from build123d import *

# Parameters (mm, degrees)
BOSS_EXTRUDE2_DEPTH = 2
SKETCH8_R           = 0.46
CUT_EXTRUDE1_DEPTH  = 6.857687257
CUT_EXTRUDE3_DEPTH  = 5.308421985
BOSS_EXTRUDE3_DEPTH = 0.75
SKETCH11_W          = 5.5
SKETCH11_H          = 5
BOSS_EXTRUDE4_DEPTH = 0.75
FILLET1_R           = 2
CUT_EXTRUDE5_DEPTH  = 1.75
SKETCH13_W          = 0.75
SKETCH13_H          = 1.75
CUT_EXTRUDE4_DEPTH  = 0.5
FILLET2_R           = 0.25
FILLET3_R           = 0.25
SKETCH15_RX         = 1.5
SKETCH15_RY         = 0.25
CUT_EXTRUDE6_DEPTH  = 10


with BuildPart() as part:
    # Sketch5 → Boss-Extrude2 (new body)
    with BuildSketch(Plane(origin=(0, 0, 0), x_dir=(1, 0, 0), z_dir=(0, 1, 0))):
        Polygon((-2.25, -2), (1.75, -2), (3.25, -2), (3.25, 2), (1.75, 2), (-2.25, 2), align=None)
    extrude(amount=-BOSS_EXTRUDE2_DEPTH)

    # Sketch8 → Cut-Extrude1 (cut, through all)
    with BuildSketch(Plane(origin=(0.85, 2.55, 0), x_dir=(0.948683298050514, -0.3162277660168378, 0), z_dir=(0.3162277660168378, 0.948683298050514, 0))):
        with Locations((1.829822128, 0)):
            Circle(SKETCH8_R)
    extrude(amount=-CUT_EXTRUDE1_DEPTH, mode=Mode.SUBTRACT)

    # Sketch12 → Cut-Extrude3 (cut, through all)
    with BuildSketch(Plane(origin=(0, 0, 0), x_dir=(1, 0, 0), z_dir=(0, 1, 0))):
        Polygon((-1.5, 1.25), (-1.5, -1.25), (-0.75, -1.25), (0, 0), (-0.75, 1.25), align=None)
    extrude(amount=-CUT_EXTRUDE3_DEPTH, mode=Mode.SUBTRACT)

    # Sketch10 → Boss-Extrude3 (add)
    with BuildSketch(Plane.XY.offset(2)):
        Polygon((3.25, -2), (3.25, 3), (-2.25, 3), (-2.25, 0), (-2.25, -2), align=None)
    boss_extrude3 = extrude(amount=BOSS_EXTRUDE3_DEPTH)

    # Mirror1: Boss-Extrude3 across plane
    add(boss_extrude3.mirror(Plane.XY))

    # Sketch11 → Boss-Extrude4 (add)
    with BuildSketch(Plane(origin=(3.25, 0, 0), x_dir=(0, 0, -1), z_dir=(1, 0, 0))):
        with Locations((0, 0.5)):
            Rectangle(SKETCH11_W, SKETCH11_H)
    extrude(amount=BOSS_EXTRUDE4_DEPTH)

    # Fillet1
    fillet1_edges = [part.edges().sort_by_distance(p)[0] for p in [
        (-2.25, 3, 2.375),
        (-2.25, 3, -2.375),
    ]]
    fillet(fillet1_edges, radius=FILLET1_R)

    # Sketch14 → Cut-Extrude5 (cut)
    with BuildSketch(Plane.XZ.offset(2)):
        Polygon((-2.25, 2.75), (-2.25, 2.25), (3.5, 2.25), (3.5, -2.25), (-2.25, -2.25), (-2.25, -2.75), (4, -2.75), (4, 2.75), align=None)
    extrude(amount=-CUT_EXTRUDE5_DEPTH, mode=Mode.SUBTRACT)

    # Sketch13 → Cut-Extrude4 (cut)
    with BuildSketch(Plane.XY.offset(2.25)):
        with Locations((-0.5, -1.125)):
            Rectangle(SKETCH13_W, SKETCH13_H)
        with Locations((2.25, -1.125)):
            Rectangle(SKETCH13_W, SKETCH13_H)
    cut_extrude4 = extrude(amount=-CUT_EXTRUDE4_DEPTH, mode=Mode.SUBTRACT)

    # Mirror2: Cut-Extrude4 across plane
    add(cut_extrude4.mirror(Plane.XY), mode=Mode.SUBTRACT)

    # Fillet2
    fillet2_edges = [part.edges().sort_by_distance(p)[0] for p in [
        (3.0625, -0.25, -2.25),
        (3.5, -0.25, 0),
        (3.5, -1.125, -2.25),
        (-1.5625, -0.25, 2.25),
        (0.875, -0.25, 2.25),
        (3.0625, -0.25, 2.25),
        (0.875, -0.25, -2.25),
        (-1.5625, -0.25, -2.25),
    ]]
    fillet(fillet2_edges, radius=FILLET2_R)

    # Fillet3
    fillet3_edges = [part.edges().sort_by_distance(p)[0] for p in [
        (4, 1.375, -2.75),
        (4, 1.375, 2.75),
    ]]
    fillet(fillet3_edges, radius=FILLET3_R)

    # Sketch15 → Cut-Extrude6 (cut)
    with BuildSketch(Plane(origin=(4, 0, 0), x_dir=(0, 0, -1), z_dir=(1, 0, 0))):
        with Locations((0, 3)):
            Ellipse(SKETCH15_RX, SKETCH15_RY)
    extrude(amount=-CUT_EXTRUDE6_DEPTH, mode=Mode.SUBTRACT)


solid = part.part
Here's how the part is built. I have some questions about the finished solid (model axes, mm). A direction names the side the tool comes from. Round coordinates to 2 decimals unless told otherwise and drop trailing zeros. Order: outer loops, then holes, each group sorted by start corner. A loop starts at its lowest first (then second) coordinate and runs counter-clockwise, first axis right, second up. Notation, with made-up numbers: M 14,-11 L 68,-11 A23 ccw 68,21 Z; hole C 53.25,6 d4. An arc over 180 degrees is marked long. Return JSON: item names as keys, results as strings. Group by question number.
1. If we section it at B-B on x = 0.25: List the corners of the cut face in (y, z) for me, then the cut area to 3 significant figures.
2. If we section it at C-C on y = 0.5: List the corners of the cut face in (x, z) for me, then the cut area to 3 significant figures.
3. Please list where these lines run through material, in increasing order: probe 1 along Z at (x, y) = (3, 2.3); probe 2 along Z at (x, y) = (-1, -0.15); probe 3 along X at (y, z) = (-1.4, -0.15).
4. If we mould it in two halves opening along X, with no side actions, what happens to faces 1 (the face through (-1.68, 2.4, 2.38)), 2 (the face through (-0.37, -0.99, -0.62)), 3 (the face through (-0.38, -0.99, 0.63)), 4 (the face through (0.5, 0, 0))? For each: pulls with the +X half, pulls with the -X half, needs draft (parallel to the pull), parting line crosses it, or undercut.
5. If we section it at A-A on z = 2.1: List the corners of the cut face in (x, y) for me (3 decimals), then the cut area to 3 significant figures.
6. If we section it at D-D on x = -1.25: List the corners of the cut face in (y, z) for me.
7. On a 3-axis mill with a long thin cutter (end or side, diameter ignored), from which of +Z, -Z, +X, -X, +Y, -Y can I reach the whole of each face in a straight line? I mean faces 5 (the face through (3.5, -1, 0)), 6 (the face through (-2, -1, 2.25)), 7 (the face through (-2, -1, -2.25)), 8 (the face through (3.25, 2, 0)). Say none if no direction works.
8. I'm going to push flat-ended pins straight in: pin 1 Ø0.7 at (x, y) = (-1.5, -1) entering from -Z; pin 2 Ø0.8 at (y, z) = (-1.5, -2.5) entering from -X; pin 3 Ø1 at (x, y) = (3, -1) entering from +Z; pin 4 Ø0.6 at (y, z) = (-1, 2) entering from +X. Where does each tip first touch, or does it pass through?
Reply:
{
 "1": {"outline": "M -2,-2.25 L -0.5,-2.25 A0.25 cw -0.25,-2.5 L -0.25,-2.75 L 3,-2.75 L 3,-2 L 0,-2 L 0,2 L 3,2 L 3,2.75 L -0.25,2.75 L -0.25,2.5 A0.25 cw -0.5,2.25 L -2,2.25 Z", "area": "13.8 mm^2"},
 "2": {"outline": "M -2.25,-2.75 L 3.75,-2.75 A0.25 ccw 4,-2.5 L 4,2.5 A0.25 ccw 3.75,2.75 L -2.25,2.75 L -2.25,2 L 3.25,2 L 3.25,-2 L -2.25,-2 Z", "area": "12.3 mm^2"},
 "3": {"probe 1": "-2.75 to -2, 2 to 2.75", "probe 2": "-2.75 to -1.25, 1.25 to 2.75", "probe 3": "-2.25 to -1.5, -0.09 to 1, 1.92 to 3.5"},
 "4": {"face 1": "pulls with the -X half", "face 2": "undercut", "face 3": "undercut", "face 4": "needs draft"},
 "5": {"outline": "M -2.25,-2 L -0.875,-2 L -0.875,-0.25 L -0.125,-0.25 L -0.125,-2 L 1.875,-2 L 1.875,-0.25 L 2.625,-0.25 L 2.625,-2 L 3.5,-2 L 3.5,-0.5 A0.25 cw 3.75,-0.25 L 4,-0.25 L 4,3 L -0.25,3 A2 ccw -2.25,1 Z", "area": "26.9 mm^2"},
 "6": {"outline": "M -2,-2.25 L -0.5,-2.25 A0.25 cw -0.25,-2.5 L -0.25,-2.75 L 2.73,-2.75 L 2.73,-2 L 0,-2 L 0,-1.25 L -2,-1.25 Z; M -2,1.25 L 0,1.25 L 0,2 L 2.73,2 L 2.73,2.75 L -0.25,2.75 L -0.25,2.5 A0.25 cw -0.5,2.25 L -2,2.25 Z"},
 "7": {"face 5": "+Z, -Z, +X, -Y", "face 6": "+Z, +X, -X, -Y", "face 7": "-Z, +X, -X, -Y", "face 8": "-X, +Y"},
 "8": {"pin 1": "z = -2.25", "pin 2": "x = -2.25", "pin 3": "z = 2.25", "pin 4": "x = 3.5"}
}
